Work out the finished part from the listing and answer in its coordinate system (mm). Face numbers are marked on the shaded views. Round coordinates to 2 decimals unless told otherwise and drop trailing zeros. Loops run counter-clockwise (first coordinate to the right, second up) from the corner with the lowest first, then second, coordinate; pieces in that order, holes last. Notation, with made-up numbers: (-18.5, 61) - (-13.5, 61) arc R16 ccw to (-13.5, 90) - close; hole circle Ø11 at (-31, 22.5). An arc over 180 degrees is marked (long way). Use CSV: the item, a comma, the result in double quotes. Start each with the question number.
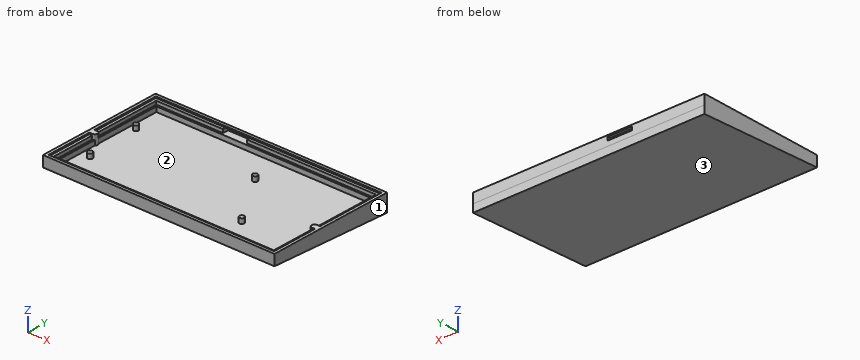
from build123d import *

# Parameters (mm, degrees)
MODEL_W             = 239.114
MODEL_H             = 131.298938207
EXTRUDE_2_DEPTH     = 10
EXTRUDE_3_DEPTH     = 8.5
EXTRUDE_4_DEPTH     = 5
SKETCH_3_R          = 2.5
EXTRUDE_5_DEPTH     = 5
EXTRUDE_5_2_DEPTH   = 5
EXTRUDE_5_3_DEPTH   = 5
EXTRUDE_5_4_DEPTH   = 5
EXTRUDE_6_DEPTH     = 239.114
SKETCH_5_W          = 25
SKETCH_5_H          = 5.998631207
CUT_EXTRUDE_1_DEPTH = 3.5


with BuildPart() as part:
    # Model → Extrude 2 (new body)
    with BuildSketch(Plane.XY):
        with Locations((559.31883528, 226.885059923)):
            Rectangle(MODEL_W, MODEL_H)
        with BuildLine():
            Line((442.76183528, 289.535897819), (675.87583528, 289.535897819))
            Line((675.87583528, 289.535897819), (675.87583528, 217.861297819))
            Line((675.87583528, 217.861297819), (672.87583528, 217.861297819))
            ThreePointArc((672.87583528, 217.861297819), (671.805369011, 217.663814896), (670.87583528, 217.097365797))
            ThreePointArc((670.87583528, 217.097365797), (669.87583528, 214.861297819), (670.87583528, 212.625229842))
            ThreePointArc((670.87583528, 212.625229842), (671.805369011, 212.058780742), (672.87583528, 211.861297819))
            Line((672.87583528, 211.861297819), (675.87583528, 211.861297819))
            Line((675.87583528, 211.861297819), (675.87583528, 164.235590819))
            Line((675.87583528, 164.235590819), (442.76183528, 164.235590819))
            Line((442.76183528, 164.235590819), (442.76183528, 211.861297819))
            Line((442.76183528, 211.861297819), (445.76183528, 211.861297819))
            ThreePointArc((445.76183528, 211.861297819), (446.832301549, 212.058780742), (447.76183528, 212.625229842))
            ThreePointArc((447.76183528, 212.625229842), (448.76183528, 214.861297819), (447.76183528, 217.097365797))
            ThreePointArc((447.76183528, 217.097365797), (446.832301549, 217.663814896), (445.76183528, 217.861297819))
            Line((445.76183528, 217.861297819), (442.76183528, 217.861297819))
            Line((442.76183528, 217.861297819), (442.76183528, 289.535897819))
        make_face(mode=Mode.SUBTRACT)
    extrude(amount=EXTRUDE_2_DEPTH)

    # Model_4 → Extrude 3 (add)
    with BuildSketch(Plane.XY):
        Polygon((445.76183528, 167.235590819), (445.76183528, 211.861297819), (442.76183528, 211.861297819), (442.76183528, 164.235590819), (675.87583528, 164.235590819), (675.87583528, 211.861297819), (672.87583528, 211.861297819), (672.87583528, 167.235590819), align=None)
        Polygon((442.76183528, 217.861297819), (442.76183528, 289.535897819), (675.87583528, 289.535897819), (675.87583528, 217.861297819), (672.87583528, 217.861297819), (672.87583528, 286.535897819), (445.76183528, 286.535897819), (445.76183528, 217.861297819), align=None)
    extrude(amount=EXTRUDE_3_DEPTH)

    # Model_5 → Extrude 4 (add)
    with BuildSketch(Plane.XY):
        with BuildLine():
            ThreePointArc((672.87583528, 211.861297819), (671.805369011, 212.058780742), (670.87583528, 212.625229842))
            Line((670.87583528, 212.625229842), (670.87583528, 169.235590819))
            Line((670.87583528, 169.235590819), (447.76183528, 169.235590819))
            Line((447.76183528, 169.235590819), (447.76183528, 212.625229842))
            ThreePointArc((447.76183528, 212.625229842), (446.832301549, 212.058780742), (445.76183528, 211.861297819))
            Line((445.76183528, 211.861297819), (445.76183528, 167.235590819))
            Line((445.76183528, 167.235590819), (672.87583528, 167.235590819))
            Line((672.87583528, 167.235590819), (672.87583528, 211.861297819))
        make_face()
        with BuildLine():
            ThreePointArc((670.87583528, 217.097365797), (671.805369011, 217.663814896), (672.87583528, 217.861297819))
            Line((672.87583528, 217.861297819), (672.87583528, 286.535897819))
            Line((672.87583528, 286.535897819), (539.76183528, 286.535897819))
            Line((539.76183528, 286.535897819), (514.76183528, 286.535897819))
            Line((514.76183528, 286.535897819), (445.76183528, 286.535897819))
            Line((445.76183528, 286.535897819), (445.76183528, 217.861297819))
            ThreePointArc((445.76183528, 217.861297819), (446.832301549, 217.663814896), (447.76183528, 217.097365797))
            Line((447.76183528, 217.097365797), (447.76183528, 284.535897819))
            Line((447.76183528, 284.535897819), (670.87583528, 284.535897819))
            Line((670.87583528, 284.535897819), (670.87583528, 217.097365797))
        make_face()
    extrude(amount=EXTRUDE_4_DEPTH)



with BuildPart() as body_2:
    # Sketch 3 → Extrude 5 (new body)
    with BuildSketch(Plane(origin=(0, 0, 0), x_dir=(-1, 0, 0), z_dir=(0, 0, -1))):
        with Locations((-577.62472278, 252.961297819)):
            Circle(SKETCH_3_R)
    extrude(amount=-EXTRUDE_5_DEPTH)


with BuildPart() as body_3:
    # Sketch 3 → Extrude 5 2 (new body)
    with BuildSketch(Plane(origin=(0, 0, 0), x_dir=(-1, 0, 0), z_dir=(0, 0, -1))):
        with Locations((-614.53372278, 195.811572819)):
            Circle(SKETCH_3_R)
    extrude(amount=-EXTRUDE_5_2_DEPTH)


with BuildPart() as body_4:
    # Sketch 3 → Extrude 5 3 (new body)
    with BuildSketch(Plane(origin=(0, 0, 0), x_dir=(-1, 0, 0), z_dir=(0, 0, -1))):
        with Locations((-457.84983528, 195.811597819)):
            Circle(SKETCH_3_R)
    extrude(amount=-EXTRUDE_5_3_DEPTH)


with BuildPart() as body_5:
    # Sketch 3 → Extrude 5 4 (new body)
    with BuildSketch(Plane(origin=(0, 0, 0), x_dir=(-1, 0, 0), z_dir=(0, 0, -1))):
        with Locations((-454.62472278, 252.961297819)):
            Circle(SKETCH_3_R)
    extrude(amount=-EXTRUDE_5_4_DEPTH)


with BuildPart() as part_1:
    add(part.part)

    add(body_2.part)  # Extrude 6 merges body 2

    add(body_3.part)  # Extrude 6 merges body 3

    add(body_4.part)  # Extrude 6 merges body 4

    add(body_5.part)  # Extrude 6 merges body 5
    # Sketch 4 → Extrude 6 (add)
    with BuildSketch(Plane.ZY.offset(-439.76183528)):
        Polygon((-7.881170053, 292.536137164), (-1, 161.235590819), (0, 161.235590819), (0, 292.534529026), align=None)
    extrude(amount=-EXTRUDE_6_DEPTH)

    # Sketch 5 → Cut-Extrude 1 (cut)
    with BuildSketch(Plane.XY.offset(8.5)):
        with Locations((527.26183528, 289.535213423)):
            Rectangle(SKETCH_5_W, SKETCH_5_H)
    extrude(amount=-CUT_EXTRUDE_1_DEPTH, mode=Mode.SUBTRACT)


solid = part_1.part
Item 1: The mould has two halves that part along Y. Classify the marked faces 1, 2 and 3: pulls with the +Y half, pulls with the -Y half, needs draft (parallel to the pull), parting line crosses it, or undercut.
Item 2: Each of these flat-tipped pins is pushed along its axis until it touches: pin 1 Ø5.5 at (x, y) = (456.5, 196.5) entering from +Z; pin 2 Ø1.5 at (x, y) = (532, 241) entering from -Z; pin 3 Ø5 at (x, z) = (655, -3) entering from -Y; pin 4 Ø0.9 at (x, y) = (523.5, 291.5) entering from -Z. Where does it stop, or does it pass through?
Item 3: A cutting plane is placed at B-B (x = 582.5). Determine the outline of the cut face in (y, z).
Item 4: A cutting plane is placed at C-C (y = 179). Determine the outline of the cut face in (x, z), plus the area to 3 significant figures.
Item 5: A cutting plane is placed at D-D (z = -3.5). Determine the outline of the cut face in (x, y), plus the area to 3 significant figures.
Item 6: A cutting plane is placed at A-A (x = 519). Determine the outline of the cut face in (y, z).
Item 7: Find the intervals of material crossed by probe 1 along Y at (x, z) = (464.5, 4.25); probe 2 along X at (y, z) = (252, 7.5); probe 3 along X at (y, z) = (281, 0.5), in increasing order. Write a range as [from, to].
Result sheet:
1,face 1,"needs draft"
1,face 2,"undercut"
1,face 3,"pulls with the -Y half"
2,pin 1,"z = 5"
2,pin 2,"z = -5.22"
2,pin 3,"y = 161.24"
2,pin 4,"z = -7.85"
3,outline,"(161.24, -1) - (292.54, -7.88) - (292.53, 0) - (292.53, 10) - (289.54, 10) - (289.54, 8.5) - (286.54, 8.5) - (286.54, 5) - (284.54, 5) - (284.54, 0) - (169.24, 0) - (169.24, 5) - (167.24, 5) - (167.24, 8.5) - (164.24, 8.5) - (164.24, 10) - (161.24, 10) - close"
4,outline,"(439.76, -1.93) - (678.88, -1.93) - (678.88, 10) - (675.88, 10) - (675.88, 8.5) - (672.88, 8.5) - (672.88, 5) - (670.88, 5) - (670.88, 0) - (447.76, 0) - (447.76, 5) - (445.76, 5) - (445.76, 8.5) - (442.76, 8.5) - (442.76, 10) - (439.76, 10) - close"
4,area,"593 mm^2"
5,outline,"(439.76, 208.94) - (678.88, 208.94) - (678.88, 292.54) - (439.76, 292.54) - close"
5,area,"20,000 mm^2"
6,outline,"(161.24, -1) - (292.54, -7.88) - (292.53, 0) - (292.53, 5) - (284.54, 5) - (284.54, 0) - (169.24, 0) - (169.24, 5) - (167.24, 5) - (167.24, 8.5) - (164.24, 8.5) - (164.24, 10) - (161.24, 10) - close; (289.54, 8.5) - (292.53, 8.5) - (292.53, 10) - (289.54, 10) - close"
7,probe 1,"[161.24, 169.24], [284.54, 292.53]"
7,probe 2,"[439.76, 445.76], [672.88, 678.88]"
7,probe 3,"[439.76, 447.76], [670.88, 678.88]"
